CAD build for the part. Positions are in the model's coordinates, mm. Face numbers are marked on the shaded views. A direction names the side the tool comes from. Give positions to 0.01 mm unless a question says otherwise; leave off trailing zeros. Write each loop counter-clockwise with the first axis right and the second up, starting at its lowest first coordinate (ties: lowest second). Pieces come first, ordered by that corner, then holes. Notation, with made-up numbers: (-6, 52) - (6, 52) arc R10 ccw to (6, 64) - close; hole circle Ø6 at (59.25, 61.5). An arc over 180 degrees is marked (long way). Put each result on its own line as item: value. Start each with the question number.
1. Cut at B-B on y = -94. List the corners of the cut face in (x, z).
2. Tool access for the marked faces 1 and 2: list every direction of +Z, -Z, +X, -X, +Y, -Y with a clear straight run to the whole face (end or side of a thin tool).
3. Wall check: line 1 (X direction, y = -191.75, z = 0); line 2 (Y direction, x = 51.5, z = -143.5); line 3 (X direction, y = 152.75, z = 0). Give the ranges that are in metal, low to high.
4. Drop flat-ended pins along their axis: pin 1 (1 mm diameter, centred on x = 104.5, z = -36.5, fed in from +Y); pin 2 (3 mm diameter, centred on x = 122, y = 6.5, fed in from -Z); pin 3 (1.5 mm diameter, centred on x = -75, y = 113, fed in from -Z). Give the stop position or say it passes through.
5. Cut at A-A on y = 74. List the corners of the cut face in (x, z).
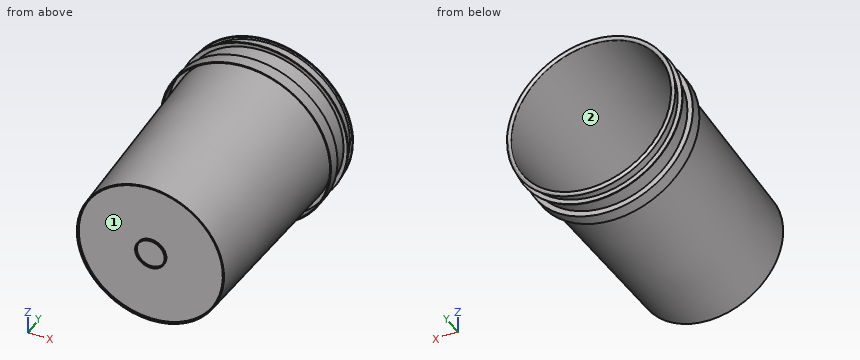
from build123d import *

# Parameters (mm, degrees)
SCALE1_SCALE = 24.694444444


with BuildPart() as part:
    # Sketch1 → Revolve1 (revolve)
    with BuildSketch(Plane.XY, mode=Mode.PRIVATE) as revolve1_sk:
        with BuildLine():
            Line((0, -0.094227964), (-1.061247893, -0.094227964))
            Line((-1.061247893, -0.094227964), (-1.061247893, -0.200590652))
            Line((-1.061247893, -0.200590652), (-1.13806539, -0.200590652))
            Line((-1.13806539, -0.200590652), (-1.13806539, -0.094227964))
            Line((-1.13806539, -0.094227964), (-5.395815038, -0.08834647))
            Line((-5.395815038, -0.08834647), (-5.395815038, -0.200590652))
            Line((-5.395815038, -0.200590652), (-5.482893557, -0.200590652))
            Line((-5.482893557, -0.200590652), (-5.966284415, 14.474501006))
            Line((-5.966284415, 14.474501006), (-6.27388996, 14.425226712))
            Line((-6.27388996, 14.425226712), (-6.27388996, 13.549490193))
            Line((-6.27388996, 13.549490193), (-6.346091135, 13.549490193))
            Line((-6.346091135, 13.549490193), (-6.346091135, 14.485650511))
            Line((-6.346091135, 14.485650511), (-5.968643269, 14.546112611))
            Line((-5.968643269, 14.546112611), (-6.016345654, 15.994292405))
            Line((-6.016345654, 15.994292405), (-6.340619476, 15.947459591))
            Line((-6.340619476, 15.947459591), (-6.350120653, 16.013246438))
            Line((-6.350120653, 16.013246438), (-6.025480097, 16.060132217))
            Line((-6.025480097, 16.060132217), (-6.048293639, 16.861870002))
            ThreePointArc((-6.048293639, 16.861870002), (-6.138820306, 16.886263059), (-6.215951685, 16.832963442))
            Line((-6.215951685, 16.832963442), (-6.256868902, 16.832963442))
            ThreePointArc((-6.256868902, 16.832963442), (-6.123324966, 17.009958484), (-5.954407696, 16.866333335))
            Line((-5.954407696, 16.866333335), (-5.39906689, 0.006938679))
            Line((-5.39906689, 0.006938679), (0, 0))
            Line((0, 0), (0, -0.094227964))
        make_face()
    revolve(revolve1_sk.sketch.rotate(Axis((0, 0, 0), (0, 1, 0)), 270), axis=Axis((0, 0, 0), (0, 1, 0)))


with BuildPart() as part_1:
    # Scale1: scaled about (0, 7.960069981, 0)
    add(part.part.scale(SCALE1_SCALE).moved(Location((0, -188.609435939, 0))))


solid = part_1.part
Report:
1. outline: circle Ø277.35 at (0, 0); hole circle Ø272.88 at (0, 0)
2. face 1: -Y
2. face 2: +Y
3. line 1: x = -135.46 to -133.25, -28.1 to -26.21, 26.21 to 28.1, 133.25 to 135.46
3. line 2: y = 168.01 to 169.79, 205.8 to 207.46, 228.08 to 231.08
3. line 3: x = -156.71 to -154.93, -146.8 to -144.57, 144.57 to 146.8, 154.93 to 156.71
4. pin 1: stops at y = -188.47
4. pin 2: stops at z = -75.1
4. pin 3: stops at z = -125.12
5. outline: circle Ø288.42 at (0, 0); hole circle Ø283.94 at (0, 0)
